Geometry check sheet. Reference: the model listing, model coordinates, mm. A direction names the side the tool comes from. Give positions to 0.01 mm unless a question says otherwise; leave off trailing zeros. Order: outer loops, then holes, each group sorted by start corner. A loop starts at its lowest first (then second) coordinate and runs counter-clockwise, first axis right, second up. Notation, with made-up numbers: (60, 4) - (93, 4) arc R5 cw to (93, 12) - close; hole circle Ø7 at (-27.75, 11.5). An arc over 180 degrees is marked (long way). Put each result on its own line as item: value. Start each with the question number.
```python
from build123d import *

# Parameters (mm, degrees)
SKETCH1_W           = 45.8
SKETCH1_H           = 39.7
BOSS_EXTRUDE1_DEPTH = 24.9
SKETCH2_W           = 21.252664268
SKETCH2_H           = 4.1
CUT_EXTRUDE1_DEPTH  = 24.9
SKETCH3_R           = 5.707882507
BOSS_EXTRUDE2_DEPTH = 20
SKETCH4_R           = 5.223999668
BOSS_EXTRUDE3_DEPTH = 20
BOSS_EXTRUDE4_DEPTH = 10
BOSS_EXTRUDE5_DEPTH = 20
SKETCH7_R           = 2.5
CUT_EXTRUDE2_DEPTH  = 100


with BuildPart() as part:
    # Sketch1 → Boss-Extrude1 (new body)
    with BuildSketch(Plane.XY):
        with Locations((-66.792592593, 34.14526749)):
            Rectangle(SKETCH1_W, SKETCH1_H)
    extrude(amount=BOSS_EXTRUDE1_DEPTH)

    # Sketch2 → Cut-Extrude1 (cut)
    with BuildSketch(Plane.XY.offset(24.9)):
        with Locations((-54.518924727, 51.94526749)):
            Rectangle(SKETCH2_W, SKETCH2_H)
    extrude(amount=-CUT_EXTRUDE1_DEPTH, mode=Mode.SUBTRACT)

    # Sketch3 → Boss-Extrude2 (add)
    with BuildSketch(Plane(origin=(0, 53.99526749, 0), x_dir=(1, 0, 0), z_dir=(0, 1, 0))):
        with Locations((-74.419404391, -12.144927528)):
            Circle(SKETCH3_R)
    extrude(amount=BOSS_EXTRUDE2_DEPTH)

    # Sketch4 → Boss-Extrude3 (add)
    with BuildSketch(Plane(origin=(0, 49.89526749, 0), x_dir=(1, 0, 0), z_dir=(0, 1, 0))):
        with Locations((-55.701029149, -13.081935835)):
            Circle(SKETCH4_R)
    extrude(amount=BOSS_EXTRUDE3_DEPTH)

    # Sketch5 → Boss-Extrude4 (add)
    with BuildSketch(Plane.ZY.offset(89.692592593)):
        Polygon((18.845976306, 21.012997096), (18.845976306, 28.313544296), (12.523516969, 31.963817896), (6.201057632, 28.313544296), (6.201057632, 21.012997096), (12.523516969, 17.362723496), align=None)
    extrude(amount=BOSS_EXTRUDE4_DEPTH)

    # Sketch6 → Boss-Extrude5 (add)
    with BuildSketch(Plane(origin=(-43.892592593, 0, 0), x_dir=(0, 0, -1), z_dir=(1, 0, 0))):
        Polygon((-17.449153894, 30.618145188), (-12.514917778, 33.466927738), (-12.514917778, 39.164492838), (-17.449153894, 42.013275388), (-22.383390011, 39.164492838), (-22.383390011, 33.466927738), align=None)
        Polygon((-7.414087621, 16.686679556), (-2.60718663, 19.461945137), (-2.60718663, 25.012476299), (-7.414087621, 27.78774188), (-12.220988612, 25.012476299), (-12.220988612, 19.461945137), align=None)
    extrude(amount=BOSS_EXTRUDE5_DEPTH)

    # Sketch7 → Cut-Extrude2 (cut)
    with BuildSketch(Plane.XY.offset(24.9)):
        with Locations((-67.30075544, 18.790910281)):
            Circle(SKETCH7_R)
        with Locations((-86.236984796, 50.57800228)):
            Circle(SKETCH7_R)
        with Locations((-49.59462681, 45.445985012)):
            Circle(SKETCH7_R)
    extrude(amount=-CUT_EXTRUDE2_DEPTH, mode=Mode.SUBTRACT)


solid = part.part
```
Item 1: Cross-section at B-B (z = 21.25). Enter the section's corners in (x, y), and give its area (3 significant figures).
Item 2: Gauge pin test, flat ends, axial feed: pin 1 Ø6 at (x, y) = (-97, 25.5) entering from +Z; pin 2 Ø1.7 at (x, y) = (-37.5, 36.5) entering from +Z; pin 3 Ø2 at (y, z) = (41, 10.5) entering from -X; pin 4 Ø8 at (x, y) = (-49.59, 45.45) entering from -Z. Record the tip position at first contact, or that the pin passes through.
Item 3: Cross-section at A-A (y = 24). Enter the section's corners in (x, z).
Item 4: Cross-section at D-D (y = 67.5). Enter the section's corners in (x, z).
Item 5: Release check for a two-part mould opening along X. For faces 6 (the face through (-34, 40.6, 19.9)), 7 (the face through (-43.893, 32, 12)), 8 (the face through (-69.8, 18.9, 12.6)) record: +X half, -X half, draft (parallel to the pull), parting line (faces both ways), or undercut.
Item 6: Cross-section at C-C (x = -76). Enter the section's corners in (y, z), and give its area (3 significant figures).
Item 7: Thickness scan on line 1 along X through (y, z) = (50.5, 21.5); line 2 along X through (y, z) = (19, 13.5); line 3 along X through (y, z) = (48, 23). Record the ranges inside material, lowest first.
Item 8: Set-up check for faces 1 (the face through (-60.92, 59.76, 12.85)), 2 (the face through (-34.033, 18.055, 5.044)), 3 (the face through (-34, 22, 2.607)), 4 (the face through (-34.03, 26.42, 9.78)), 5 (the face through (-95, 25, 18.846)): record each of +Z, -Z, +X, -X, +Y, -Y from which the full face is reachable in a straight line by a thin tool's end or side.
Recorded:
1. outline: (-89.69, 14.3) - (-43.89, 14.3) - (-43.89, 32.81) - (-23.89, 32.81) - (-23.89, 39.82) - (-43.89, 39.82) - (-43.89, 49.9) - (-65.15, 49.9) - (-65.15, 54) - (-89.69, 54) - close; hole circle Ø5 at (-86.24, 50.58); hole circle Ø5 at (-67.3, 18.79); hole circle Ø5 at (-49.59, 45.45)
1. area: 1,810 mm^2
2. pin 1: stops at z = 18.85
2. pin 2: stops at z = 22.38
2. pin 3: stops at x = -89.69
2. pin 4: stops at z = 0
3. outline: (-99.69, 6.2) - (-89.69, 6.2) - (-89.69, 0) - (-43.89, 0) - (-43.89, 2.61) - (-23.89, 2.61) - (-23.89, 12.22) - (-43.89, 12.22) - (-43.89, 24.9) - (-89.69, 24.9) - (-89.69, 18.85) - (-99.69, 18.85) - close
4. outline: circle Ø11.42 at (-74.42, 12.14); circle Ø10.45 at (-55.7, 13.08)
5. face 6: draft
5. face 7: +X half
5. face 8: undercut
6. outline: (14.3, 0) - (54, 0) - (54, 6.66) - (74, 6.66) - (74, 17.63) - (54, 17.63) - (54, 24.9) - (14.3, 24.9) - close
6. area: 1,210 mm^2
7. line 1: x = -89.69 to -88.74, -83.74 to -65.15
7. line 2: x = -99.69 to -69.79, -64.81 to -43.89
7. line 3: x = -89.69 to -43.89
8. face 1: +Y
8. face 2: -Z, +X, -Y
8. face 3: -Z, +X, +Y, -Y
8. face 4: +Z, +X, +Y
8. face 5: +Z, -X, +Y, -Y
